For this review, take the finished solid that the model builds, in its own axes (mm). A direction names the side the tool comes from. Give positions to 0.01 mm unless a question says otherwise; leave off trailing zeros. Loops run counter-clockwise (first coordinate to the right, second up) from the corner with the lowest first, then second, coordinate; pieces in that order, holes last. Notation, with made-up numbers: (2.25, 35.25) -> (54.25, 35.25) arc R20 ccw to (54.25, 59.25) -> close; hole circle Ø1 at (56, 75.25). An arc over 180 degrees is marked (long way). Answer as CSV lines item,"result". Start each with the question number.
Item 1: Machinability: for faces 1 (the face through (4.5, 4.5, -16)), 2 (the face through (15, -12, -10)), which of the approach directions +Z, -Z, +X, -X, +Y, -Y give a long, thin tool a straight path to every point of the face, cutting with its end or side? Answer none if there is none.
Item 2: For L1, parallel to Y at x = 0, z = -6.25; L2, parallel to Y at x = 1.5, z = -4.25; L3, parallel to Z at x = -2, y = -20, list the stretches that pass through material, from the lowest coordinate up. Write a range as from..to.
Item 3: Add section D-D on y = -20. State the section outline as (x, z) points.
Item 4: Add section A-A on y = 0. State the section outline as (x, z) points.
Item 5: Add section C-C on z = -2.75. State the section outline as (x, y) points, plus the area to 3 significant figures.
Item 6: Clearance check with flat-ended pins moving along their axes: P1, Ø1.5, axis at y = -7.5, z = -9.5, coming from the -X side; P2, Ø4, axis at y = -4, z = -14.5, coming from the -X side; P3, Ø3, axis at y = 11.5, z = -7.5, coming from the +X side. State where each tip first meets the part, or that it passes through.
Item 7: The part is to be moulded in two halves that separate along X. For faces 3 (the face through (0, -8, 0)), 4 (the face through (6, 0, -8)), 5 (the face through (-8.767, 16.856, -12.958)), say which applies: +X half, -X half, draft (parallel to the pull), parting line (faces both ways), or undercut.
Autodesk Inventor part; units mm, degrees
ref_plane "YZ Plane" through (0, 0, 0) normal (1, 0, 0) x (0, 1, 0)
ref_plane "XZ Plane" through (0, 0, 0) normal (0, 1, 0) x (-1, 0, 0)
ref_plane "XY Plane" through (0, 0, 0) normal (0, 0, 1) x (1, 0, 0)
sketch "Skizze3" plane through (0, 0, 0) normal (0, 1, 0) x (-1, 0, 0)
  line L0 (0, 0) -> (0, -18.1445)
  line L1 (6, 0) -> (6, -16)
  line L2 (6, -16) -> (19, -16)
  line L3 (19, -16) -> (19, -10)
  line L4 (19, -10) -> (22.5, -10)
  line L5 (22.5, -10) -> (22.5, 0)
  line L6 (22.5, 0) -> (19, 0)
  line L7 (19, 0) -> (19, -0.5)
  line L8 (19, -0.5) -> (18, 0)
  line L9 (18, 0) -> (6, 0)
  point P0 (19, -0.25)
  dimension "d4" = 16
  dimension "d5" = 10
  dimension "d6" = 12
  dimension "d7" = 38
  dimension "d8" = 45
  dimension "d9" = 1
  dimension "d10" = 0.5
revolve "Umdrehung1" add sketch "Skizze3" angle 360 about axis through (0, 0, 0) along (0, 0, -1)
properties part number "BT602_trajan20_21"
Computed values:
1,face 1,"-Z, +X, -X, +Y, -Y"
1,face 2,"-Z"
2,L1,"-22.5..-6, 6..22.5"
2,L2,"-22.45..-5.81, 5.81..22.45"
2,L3,"-10..0"
3,outline,"(-10.31, -10) -> (10.31, -10) -> (10.31, 0) -> (-10.31, 0) -> close"
4,outline,"(-22.5, -10) -> (-19, -10) -> (-19, -16) -> (-6, -16) -> (-6, 0) -> (-18, 0) -> (-19, -0.5) -> (-19, 0) -> (-22.5, 0) -> close; (6, -16) -> (19, -16) -> (19, -10) -> (22.5, -10) -> (22.5, 0) -> (19, 0) -> (19, -0.5) -> (18, 0) -> (6, 0) -> close"
5,outline,"circle Ø45 at (0, 0); hole circle Ø12 at (0, 0)"
5,area,"1,480 mm²"
6,P1,"x = -21.46"
6,P2,"x = -18.89"
6,P3,"x = 20.16"
7,face 3,"draft"
7,face 4,"undercut"
7,face 5,"parting line"
